```python
from build123d import *

# Parameters (mm, degrees)
F1_DEPTH = 4
F2_W     = 39.9907242665
F2_H     = 8
F2_W_2   = 40.1504870662
F3_DEPTH = 4
F4_DEPTH = 4
F6_DEPTH = 101


with BuildPart() as f1:
    # F0 (on Top) → F1 (new body)
    with BuildSketch(Plane.XY):
        Polygon((-123.9547070274, -15), (123.9547070274, -15), (123.9547070274, -7), (-36.0452929726, -7), (-36.0452929726, -4), (84.0192064643, -4), (84.0192064643, 4), (83.9637443423, 4), (83.9547070274, 4), (-36.0452929726, 4), (-36.0452929726, 7), (123.9547070274, 7), (123.9547070274, 15), (-123.9547070274, 15), align=None)
    extrude(amount=F1_DEPTH)

    # F2 (on face) → F3 (join)
    with BuildSketch(Plane.XY.offset(4)):
        with Locations((103.9593448941, 11)):
            Rectangle(F2_W, F2_H)
        with Locations((103.8794634943, -11)):
            Rectangle(F2_W_2, F2_H)
    extrude(amount=F3_DEPTH)

    # F2 (on face) → F4 (join)
    with BuildSketch(Plane.XY.offset(4)):
        with Locations((103.9593448941, 11)):
            Rectangle(F2_W, F2_H)
        with Locations((103.8794634943, -11)):
            Rectangle(F2_W_2, F2_H)
    extrude(amount=F4_DEPTH)

    # F5 (on face) → F6 (cut)
    with BuildSketch(Plane.XZ.offset(15)):
        with BuildLine():
            ThreePointArc((110.4547070274, 4), (110.0153671992, 5.0606601718), (108.9547070274, 5.5))
            Line((108.9547070274, 5.5), (108.9547070274, 2.5))
            ThreePointArc((108.9547070274, 2.5), (110.0153671992, 2.9393398282), (110.4547070274, 4))
        make_face()
        with BuildLine():
            Line((108.9547070274, 2.5), (108.9547070274, 5.5))
            ThreePointArc((108.9547070274, 5.5), (107.4547070274, 4), (108.9547070274, 2.5))
        make_face()
    extrude(amount=-F6_DEPTH, mode=Mode.SUBTRACT)


solid = f1.part
```
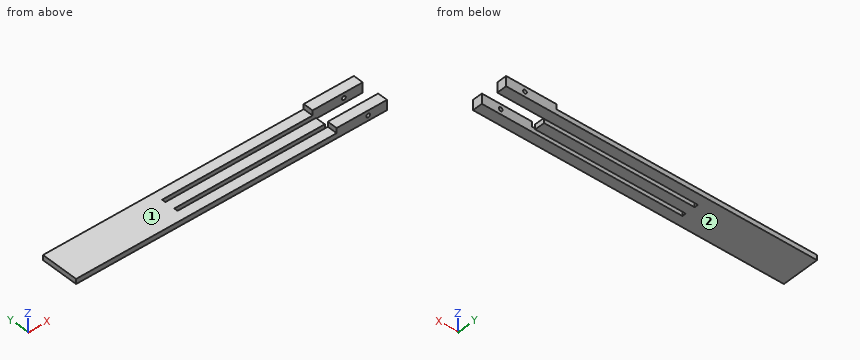
Part model, mm, in its own coordinate system. Face numbers are marked on the shaded views. A direction names the side the tool comes from. Give positions to 0.01 mm unless a question says otherwise; leave off trailing zeros. Order: outer loops, then holes, each group sorted by start corner. A loop starts at its lowest first (then second) coordinate and runs counter-clockwise, first axis right, second up. Notation, with made-up numbers: M -21.5,21 L 1.5,21 A35 cw 1.5,55 Z; hole C -33.75,65.25 d6. An arc over 180 degrees is marked long. Use a Markdown table: item, result. Add a question column.
(1) Saw through at A-A, the plane x = 78.5. Give the cut face in (y, z).
(2) Saw through at D-D, the plane x = -93. Give the cut face in (y, z), and give its area (3 significant figures).
(3) Saw through at C-C, the plane y = 12.5. Give the cut face in (x, z), and give its area (3 significant figures).
(4) Probe line 1 along Y through (x, z) = (-13, 0.5); line 2 along Y through (x, z) = (109, 6.25); line 3 along X through (y, z) = (-4.75, 2.5). List the from-to ranges inside material, lowest first. Write a range as [from, to].
(5) Saw through at B-B, the plane z = 1.25. Give the cut face in (x, y).
(6) 3-axis set-ups, long thin cutter, end or side, ignore diameter. For the marked faces 1 and 2: which of +Z, -Z, +X, -X, +Y, -Y reach the whole face in a straight line?
(7) Drop flat-ended pins along their axis: P1, Ø8, axis at x = -60.5, y = -4, coming from the +Z side; P2, Ø3, axis at y = 9.5, z = 6.5, coming from the -X side; P3, Ø2.5, axis at y = 5.5, z = 1, coming from the +X side. Give the stop position or say it passes through.
Answer key:
| question | item | result |
|---|---|---|
| 1 | outline | M -15,0 L -7,0 L -7,4 L -15,4 Z; M -4,0 L 4,0 L 4,4 L -4,4 Z; M 7,0 L 15,0 L 15,4 L 7,4 Z |
| 2 | outline | M -15,0 L 15,0 L 15,4 L -15,4 Z |
| 2 | area | 120 mm^2 |
| 3 | outline | M -123.95,0 L 123.95,0 L 123.95,8 L 83.96,8 L 83.96,4 L -123.95,4 Z; hole C 108.95,4 d3 |
| 3 | area | 1,140 mm^2 |
| 4 | line 1 | [-15, -7], [-4, 4], [7, 15] |
| 4 | line 2 | [-15, -7], [7, 15] |
| 4 | line 3 | [-123.95, -36.05] |
| 5 | outline | M -123.95,-15 L 123.95,-15 L 123.95,-7 L -36.05,-7 L -36.05,-4 L 84.02,-4 L 84.02,4 L -36.05,4 L -36.05,7 L 123.95,7 L 123.95,15 L -123.95,15 Z |
| 6 | face 1 | +Z, -X, +Y, -Y |
| 6 | face 2 | -Z, +X, -X, +Y, -Y |
| 7 | P1 | z = 4 |
| 7 | P2 | x = 83.96 |
| 7 | P3 | x = -36.05 |
